Autodesk Inventor part; units mm, degrees
ref_plane "YZ Plane" through (0, 0, 0) normal (1, 0, 0) x (0, 1, 0)
ref_plane "XZ Plane" through (0, 0, 0) normal (0, 1, 0) x (-1, 0, 0)
ref_plane "XY Plane" through (0, 0, 0) normal (0, 0, 1) x (1, 0, 0)
sketch "Náčrt1" plane through (0, 0, 0) normal (0, 1, 0) x (-1, 0, 0)
  line L0 (4.445, -2.2225) -> (4.445, -8.5725)
  line L1 (0, -8.5725) -> (0, -2.2225)
  arc A0 (0, -8.5725) -> (4.445, -8.5725) centre (2.2225, -8.5725) ccw
  arc A1 (4.445, -2.2225) -> (0, -2.2225) centre (2.2225, -2.2225) ccw
  point P0 (0, 0)
  dimension "d2" = 4.445
  dimension "d3" = 4.445
extrude "Vysunutí1" add sketch "Náčrt1" along normal blind 0.635
sketch "Náčrt2" plane through (0, 0.635, 0) normal (0, 1, 0) x (1, 0, 0)
  arc A0 (0, 8.5725) -> (-4.445, 8.5725) centre (-2.2225, 8.5725) ccw
  arc A1 (-4.445, 2.2225) -> (0, 2.2225) centre (-2.2225, 2.2225) ccw
  arc A2 (-4.1275, 2.2225) -> (-0.3175, 2.2225) centre (-2.2225, 2.2225) ccw
  arc A3 (-0.3175, 8.5725) -> (-4.1275, 8.5725) centre (-2.2225, 8.5725) ccw
  line L0 (-4.1275, 2.2225) -> (-4.1275, 8.5725)
  line L1 (-0.3175, 8.5725) -> (-0.3175, 2.2225)
  point P0 (0, 0)
  point P1 (-2.2225, 5.3975)
extrude "Vysunutí2" add sketch "Náčrt2" along normal blind 2.54
fillet "Zaoblení1" radius 0.254 4 edges at (-2.2225, 3.175, -10.4775) (-4.1275, 3.175, -5.3975) (-2.2225, 3.175, -0.3175) (-0.3175, 3.175, -5.3975)
sketch "Náčrt3" plane through (0, 0, 0) normal (0, -1, 0) x (1, 0, 0)
  circle A0 centre (-2.2225, -2.8575) radius 0.9525
  circle A1 centre (-2.2225, -7.9375) radius 0.9525
  point P0 (0, 0)
  dimension "d12" = 1.905
  dimension "d13" = 1.905
extrude "Vysunutí3" cut sketch "Náčrt3" against normal blind 0.0635
sketch "Náčrt4" plane through (-2.2225, 0.0635, -2.8575) normal (0, -1, 0) x (1, 0, 0)
  circle A0 centre (0, 0) radius 0.9525
  circle A1 centre (0, 0) radius 0.3175
  circle A2 centre (0, -5.08) radius 0.9525
  circle A3 centre (0, -5.08) radius 0.3175
  point P0 (2.2225, 2.8575)
  dimension "d16" = 0.635
extrude "Vysunutí4" add sketch "Náčrt4" along normal blind 7.62 contours A1 | A3
fillet "Zaoblení2" radius 0.254 2 edges at (-2.54, -7.5565, -2.8575) (-2.54, -7.5565, -7.9375)
properties part number "Crystal"
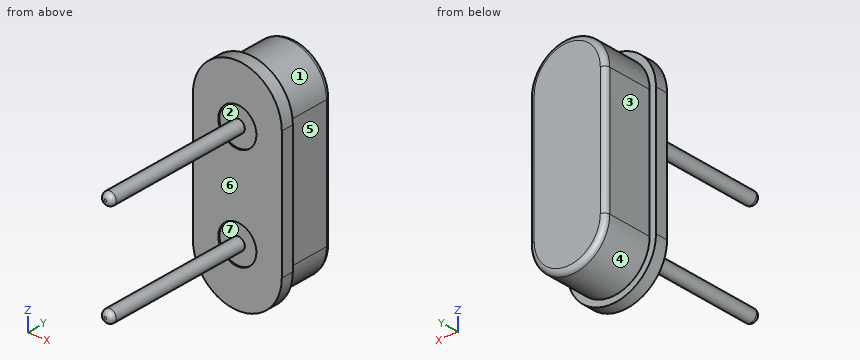
Geometry: final body of the model. Coordinates: model frame, mm. Face numbers are marked on the shaded views. A direction names the side the tool comes from. Round coordinates to 2 decimals unless told otherwise and drop trailing zeros. Order: outer loops, then holes, each group sorted by start corner. A loop starts at its lowest first (then second) coordinate and runs counter-clockwise, first axis right, second up. Notation, with made-up numbers: (23.25, 60.25) -> (59.25, 60.25) arc R6 ccw to (59.25, 69.25) -> close; hole circle Ø9 at (51.5, 73.25). An arc over 180 degrees is marked (long way). Use one line per item in the form item = value. Start each with the question number.
1. Pin query (flat end, axial travel): pin 1 Ø5 at (y, z) = (-5.5, -7) entering from +X (3 decimals); pin 2 Ø1 at (x, y) = (-3, 2) entering from -Z; pin 3 Ø1 at (x, z) = (-2.5, -8.5) entering from -Y. Return the tip coordinate at first contact, or that it passes through.
2. Cut plane B-B (y = -2.25). Return the cut outline in (x, z) (1 decimal), then the cut area to 3 significant figures.
3. Reachability of the marked faces 1, 2, 3 and 4 from +Z, -Z, +X, -X, +Y, -Y: full face, straight path, thin tool, end or side. Return the list, or none.
4. Line query: probe 1 along Y at (x, z) = (-2.7, -1.5) (3 decimals); probe 2 along Y at (x, z) = (-1.9, -8.75) (1 decimal); probe 3 along Z at (x, y) = (-3.4, 2) (3 decimals). Output: solid intervals per line, ascending.
5. Draft query along X for the marked faces 5, 6 and 7. Return one class per face: pulls with the +X half, pulls with the -X half, needs draft (parallel to the pull), parting line crosses it, or undercut.
6. Cut plane C-C (y = 1). Return the cut outline in (x, z) (1 decimal).
Solution:
q1.pin_1 = -1.905
q1.pin_2 = -10.46
q1.pin_3 = -7.55
q2.outline = circle Ø0.6 at (-2.2, -7.9); circle Ø0.6 at (-2.2, -2.9)
q2.area = 0.633 mm^2
q3.face_1 = +Z, +Y
q3.face_2 = -Y
q3.face_3 = +Z, -Z, -X, +Y
q3.face_4 = -Z, +Y
q4.probe_1 = 0 to 3.175
q4.probe_2 = 0.1 to 3.2
q4.probe_3 = -10.07 to -0.725
q5.face_5 = pulls with the +X half
q5.face_6 = needs draft
q5.face_7 = undercut
q6.outline = (-4.1, -8.6) arc R1.9 ccw to (-0.3, -8.6) -> (-0.3, -2.2) arc R1.9 ccw to (-4.1, -2.2) -> close
